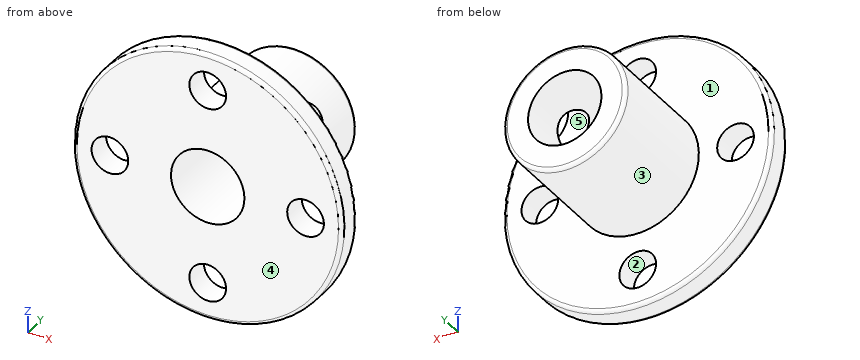
```python
from build123d import *

# Parameters (mm, degrees)
SKETCH1_R           = 5
BOSS_EXTRUDE2_DEPTH = 12
SKETCH3_R           = 11
BOSS_EXTRUDE3_DEPTH = 2
SKETCH4_R           = 3
CUT_EXTRUDE1_DEPTH  = 12
SKETCH5_R           = 1.5
CUT_EXTRUDE2_DEPTH  = 2
FILLET1_R           = 0.3
SKETCH7_R           = 1.5
CUT_EXTRUDE3_DEPTH  = 4


with BuildPart() as part:
    # Sketch1 → Boss-Extrude2 (new body)
    with BuildSketch(Plane(origin=(0, 0, 0), x_dir=(1, 0, 0), z_dir=(0, 1, 0))):
        with Locations(Location((0, 0, 0), (0, 0, 270))):
            Circle(SKETCH1_R)
    extrude(amount=BOSS_EXTRUDE2_DEPTH)

    # Sketch3 → Boss-Extrude3 (add)
    with BuildSketch(Plane(origin=(0, 0, 0), x_dir=(1, 0, 0), z_dir=(0, 1, 0))):
        with Locations(Location((0, 0, 0), (0, 0, 270))):
            Circle(SKETCH3_R)
    extrude(amount=BOSS_EXTRUDE3_DEPTH)

    # Sketch4 → Cut-Extrude1 (cut)
    with BuildSketch(Plane(origin=(0, 0, 0), x_dir=(1, 0, 0), z_dir=(0, 1, 0))):
        with Locations(Location((0, 0, 0), (0, 0, 270))):
            Circle(SKETCH4_R)
    extrude(amount=CUT_EXTRUDE1_DEPTH, mode=Mode.SUBTRACT)

    # Sketch5 → Cut-Extrude2 (cut)
    with BuildSketch(Plane(origin=(0, 2, 0), x_dir=(1, 0, 0), z_dir=(0, 1, 0))):
        with Locations(Location((0, 8, 0), (0, 0, 270))):
            Circle(SKETCH5_R)
        with Locations(Location((8, 0, 0), (0, 0, 270))):
            Circle(SKETCH5_R)
        with Locations(Location((0, -8, 0), (0, 0, 270))):
            Circle(SKETCH5_R)
        with Locations(Location((-8, 0, 0), (0, 0, 270))):
            Circle(SKETCH5_R)
    extrude(amount=-CUT_EXTRUDE2_DEPTH, mode=Mode.SUBTRACT)

    # Fillet1
    fillet1_edges = [part.edges().sort_by_distance(p)[0] for p in [
        (0, 12, -5),
        (0, 0, -11),
        (0, 2, -11),
    ]]
    fillet(fillet1_edges, radius=FILLET1_R)

    # Sketch7 → Cut-Extrude3 (cut)
    with BuildSketch(Plane(origin=(4.0625, 0, 2.914805954), x_dir=(0.5829611908180293, 0, -0.8125000000000155), z_dir=(0.8125000000000155, 0, 0.5829611908180293))):
        with Locations((0, 7)):
            Circle(SKETCH7_R)
    extrude(amount=-CUT_EXTRUDE3_DEPTH, mode=Mode.SUBTRACT)


solid = part.part
```
For this review, take the finished solid that the model builds, in its own axes (mm). Face numbers are marked on the shaded views. A direction names the side the tool comes from. Coordinates: 2 decimals unless noted, no trailing zeros. Order: outer loops, then holes, each group sorted by start corner. A loop starts at its lowest first (then second) coordinate and runs counter-clockwise, first axis right, second up. Notation, with made-up numbers: (0, 21.25) -> (50, 21.25) arc R18 ccw to (50, 44.25) -> close; hole circle Ø10 at (37.5, 52.5). An arc over 180 degrees is marked (long way). Use CSV: the item, a comma, the result in double quotes. Start each with the question number.
Item 1: Insertion check: pin 1 (5 mm diameter, centred on x = 8.5, z = -5, fed in from +Y); pin 2 (2.5 mm diameter, centred on x = 8, z = 0, fed in from +Y). Each pin has a flat end and moves straight along its axis. Give the tip position at first contact, or say it passes through.
Item 2: For the marked faces 1 and 2, list the 3-axis set-ups (+Z, -Z, +X, -X, +Y, -Y) from which the entire face can be reached by the end or side of a thin tool; tool diameter is ignored.
Item 3: We need section C-C, the plane y = 9.5. Give the boundary of the cut face in (x, z).
Item 4: We need section A-A, the plane z = 0. Give the boundary of the cut face in (x, y), then the cut area to 3 significant figures.
Item 5: Draft analysis for pull direction X (two halves, no side actions). For the marked faces 3, 4 and 5, state which applies: pulls with the +X half, pulls with the -X half, needs draft (parallel to the pull), parting line crosses it, or undercut.
Item 6: We need section D-D, the plane y = 7.5. Give the boundary of the cut face in (x, z), then the cut area to 3 significant figures.
Item 7: Wall thickness on probe 1 along X at (y, z) = (8.25, 0); probe 2 along Y at (x, z) = (8.75, -5.75); probe 3 along Z at (x, y) = (-6.75, 1.75): over which ranges is each line inside the solid? List them lowest first.
Item 8: We need section B-B, the plane x = 0.5. Give the number of separate pieces and of enclosed holes in the cut face, then the cut area to 3 significant figures.
Derived:
1,pin 1,"stops at y = 2"
1,pin 2,"passes through"
2,face 1,"+Y"
2,face 2,"+Y, -Y"
3,outline,"circle Ø10 at (0, 0); hole circle Ø6 at (0, 0)"
4,outline,"(-11, 0.3) arc R0.3 ccw to (-10.7, 0) -> (-9.5, 0) -> (-9.5, 2) -> (-10.7, 2) arc R0.3 ccw to (-11, 1.7) -> close; (-6.5, 0) -> (-3, 0) -> (-3, 12) -> (-4.7, 12) arc R0.3 ccw to (-5, 11.7) -> (-5, 2) -> (-6.5, 2) -> close; (3, 0) -> (6.5, 0) -> (6.5, 2) -> (5, 2) -> (5, 11.7) arc R0.3 ccw to (4.7, 12) -> (3, 12) -> close; (9.5, 0) -> (10.7, 0) arc R0.3 ccw to (11, 0.3) -> (11, 1.7) arc R0.3 ccw to (10.7, 2) -> (9.5, 2) -> close"
4,area,"59.9 mm^2"
5,face 3,"parting line crosses it"
5,face 4,"needs draft"
5,face 5,"undercut"
6,outline,"(1.33, 2.69) -> (3.07, 3.94) arc R5 ccw (long way) to (4.72, 1.65) -> (2.97, 0.39) arc R3 cw (long way) to start"
6,area,"44.5 mm^2"
7,probe 1,"x = -5 to -3, 3 to 5"
7,probe 2,"y = 0 to 2"
7,probe 3,"z = -8.68 to -0.83, 0.83 to 8.68"
8,separate pieces,"4"
8,enclosed holes,"0"
8,area,"61.0 mm^2"
